from build123d import *

# Parameters (mm, degrees)
F0_W      = 110
F0_H      = 75
F1_DEPTH  = 55
F3_DEPTH  = 2
F5_DEPTH  = 2
F6_W      = 112
F6_H      = 28
F7_DEPTH  = 2
F8_W      = 28
F8_H      = 59
F9_DEPTH  = 2
F10_R     = 14
F11_R     = 8
F11_R_2   = 5.25
F11_R_3   = 1.25
F12_DEPTH = 2.8


with BuildPart() as f1:
    # F0 (on Top) → F1 (new body)
    with BuildSketch(Plane.XY):
        Rectangle(F0_W, F0_H)
    extrude(amount=F1_DEPTH)

    # F2 (on face) → F3 (join)
    with BuildSketch(Plane.XY.offset(55)):
        Polygon((0, -21.541595), (0, -37.5), (55, -37.5), (55, -9.5), (33, -9.5), (21, -21.541595), align=None)
        Polygon((-33, -9.5), (-55, -9.5), (-55, -37.5), (0, -37.5), (0, -21.541595), (-21, -21.541595), align=None)
    extrude(amount=F3_DEPTH)

    # F4 (on face) → F5 (join)
    with BuildSketch(Plane.YZ.offset(55)):
        Polygon((-9.5, 0), (-9.5, 55), (-9.5, 57), (-37.5, 57), (-37.5, 0), align=None)
    extrude(amount=F5_DEPTH)

    # F6 (on face) → F7 (join)
    with BuildSketch(Plane(origin=(0, 0, 0), x_dir=(1, 0, 0), z_dir=(0, 0, -1))):
        with Locations((1, 23.5)):
            Rectangle(F6_W, F6_H)
    extrude(amount=F7_DEPTH)

    # F8 (on face) → F9 (join)
    with BuildSketch(Plane(origin=(-55, 0, 0), x_dir=(0, -1, 0), z_dir=(-1, 0, 0))):
        with Locations((23.5, 27.5)):
            Rectangle(F8_W, F8_H)
    extrude(amount=F9_DEPTH)

    # F10
    f10_edges = [f1.edges().sort_by_distance(p)[0] for p in [
        (-57, -23.5, 57),
        (-55, 14, 55),
        (57, -23.5, 57),
        (55, 14, 55),
        (57, -23.5, -2),
        (55, 14, 0),
        (-55, 14, 0),
        (-57, -23.5, -2),
    ]]
    fillet(f10_edges, radius=F10_R)

    # F11 (on face) → F12 (cut)
    with BuildSketch(Plane.XY.offset(55)):
        with BuildLine():
            ThreePointArc((-19.3, 22.817289), (-27.228965, 9.98004), (-13, 15))
            ThreePointArc((-13, 15), (-14.771035, 20.01996), (-19.3, 22.817289))
        make_face()
        with BuildLine():
            ThreePointArc((-15.75, 15), (-25.27127, 11.947337), (-19.3, 19.967142))
            ThreePointArc((-19.3, 19.967142), (-16.72873, 18.052663), (-15.75, 15))
        make_face(mode=Mode.SUBTRACT)
        with BuildLine():
            ThreePointArc((-18.05, 17.7), (-18.416117, 18.583883), (-19.3, 18.95))
            ThreePointArc((-19.3, 18.95), (-20.183883, 16.816117), (-18.05, 17.7))
        make_face()
        with Locations((21, 15)):
            Circle(F11_R)
        with Locations((21, 15)):
            Circle(F11_R_2, mode=Mode.SUBTRACT)
        with Locations((22.8, 17.7)):
            Circle(F11_R_3)
    extrude(amount=-F12_DEPTH, mode=Mode.SUBTRACT)

    # F13 (on Right) → F14 (revolve)
    with BuildSketch(Plane.YZ):
        with BuildLine():
            Line((37.5, 35), (37.5, 27.5))
            Line((37.5, 27.5), (61.365487, 27.5))
            Line((61.365487, 27.5), (66.5, 27.5))
            Line((66.5, 27.5), (70.365487, 27.5))
            ThreePointArc((70.365487, 27.5), (66.903148, 31.878728), (61.844038, 29.519393))
            ThreePointArc((61.844038, 29.519393), (61.363774, 29.057593), (60.7, 29))
            Line((60.7, 29), (37.5, 35))
        make_face()
    revolve(axis=Axis((0, 52, 27.5), (0, 1, 0)))


solid = f1.part
Model file for the job. Use its own axes, mm. A direction names the side the tool comes from. Round coordinates to 2 decimals unless told otherwise and drop trailing zeros. Order: outer loops, then holes, each group sorted by start corner. A loop starts at its lowest first (then second) coordinate and runs counter-clockwise, first axis right, second up. Notation, with made-up numbers: M 82,-23 L 116,-23 A29 cw 116,14 Z; hole C -30,88 d1. An arc over 180 degrees is marked long. Write each question's results on one line, items separated by ' | '. Start each with the question number.
(1) Drop flat-ended pins along their axis: pin 1 (12 mm diameter, centred on x = 16, y = 3.5, fed in from -Z); pin 2 (3 mm diameter, centred on x = -19.3, y = 17.7, fed in from +Z); pin 3 (2 mm diameter, centred on x = 22.8, y = 17.7, fed in from +Z). Give the stop position or say it passes through.
(2) Saw through at D-D, the plane y = 54. Give the cut face in (x, z).
(3) Saw through at B-B, the plane z = 38.5. Give the cut face in (x, y).
(4) Which spindle directions (+Z, -Z, +X, -X, +Y, -Y) get a long thin tool onto all of the face, cutting with end or side? Do faces 1 (the face through (13, -9.5, -1)), 2 (the face through (-55, 14, 28)), 3 (the face through (-50.8, 14.3, 4)). Say none if no direction does.
(5) Saw through at C-C, the plane y = -12.5. Give the cut face in (x, z), then the cut area to 3 significant figures.
(6) Saw through at A-A, the plane x = -10.5. Give the cut face in (y, z), then the cut area to 3 significant figures.
(7) Probe probe 1 along Y at (x, z) = (-21, 54.2); probe 2 along Y at (x, z) = (-19.3, 53.7); probe 3 along Y at (x, z) = (27, 50). List the from-to ranges inside material, lowest first. Write a range as from..to.
(8) Two-plate mould, pull along Y, no slides. Class faces 4 (the face through (-15.8, 13.3, 52.2)), 5 (the face through (-52.8, -23.7, 2)), 6 (the face through (27.08, -15.44, 55.99)): pulls with the +Y half, pulls with the -Y half, needs draft (parallel to the pull), parting line crosses it, or undercut.
Established:
1) pin 1: stops at z = 0 | pin 2: stops at z = 55 | pin 3: stops at z = 52.2
2) outline: C 0,27.5 d6.47
3) outline: M -57,-37.5 L 57,-37.5 L 57,-9.5 L 55,-9.5 L 55,37.5 L -55,37.5 L -55,-9.5 L -57,-9.5 Z
4) face 1: +Y | face 2: +Z, -Z, -X, +Y | face 3: -Z, -X, +Y
5) outline: M -57,12 A14 ccw -43,-2 L 43,-2 A14 ccw 57,12 L 57,43 A14 ccw 43,57 L 30.01,57 L 30.01,55 L -30.01,55 L -30.01,57 L -43,57 A14 ccw -57,43 Z | area: 6,440 mm^2
6) outline: M -37.5,-2 L -9.5,-2 L -9.5,0 L 37.5,0 L 37.5,55 L -21.54,55 L -21.54,57 L -37.5,57 Z | area: 4,210 mm^2
7) probe 1: y = -37.5..7, 9.75..20.25, 23..37.5 | probe 2: y = -37.5..7.18, 10.03..16.45, 18.95..19.97, 22.82..37.5 | probe 3: y = -37.5..37.5
8) face 4: undercut | face 5: needs draft | face 6: pulls with the +Y half
